```python
from build123d import *

# Parameters (mm, degrees)
F1_DEPTH = 76.2
F2_R     = 3.175
F3_DEPTH = 6.351


with BuildPart() as f1:
    # F0 (on Front) → F1 (new body)
    with BuildSketch(Plane.XZ):
        Polygon((0, 76.2), (0, 0), (42.919317, 0), (42.919317, 6.35), (6.35, 6.35), (6.35, 76.2), align=None)
    extrude(amount=F1_DEPTH)

    # F2 (on face) → F3 (cut, through all)
    with BuildSketch(Plane.XY.offset(6.35)):
        with Locations((24.634659, -19.05)):
            Circle(F2_R)
        with Locations((24.634659, -38.1)):
            Circle(F2_R)
        with Locations((24.634659, -57.15)):
            Circle(F2_R)
    extrude(amount=-F3_DEPTH, mode=Mode.SUBTRACT)


solid = f1.part
```
Can you work these out from the model? Positions are in its coordinate system, mm. A direction names the side the tool comes from. Coordinates: 2 decimals unless noted, no trailing zeros. Loops run counter-clockwise (first coordinate to the right, second up) from the corner with the lowest first, then second, coordinate; pieces in that order, holes last. Notation, with made-up numbers: (37.5, 28) -> (70.5, 28) arc R21 cw to (70.5, 66) -> close; hole circle Ø1 at (39.5, -29.75). An arc over 180 degrees is marked (long way). Put each result on its own line as item: value. Start each with the question number.
Q1. Thinking about a two-plate mould opening in Y: for faces 3 (the face through (5, 0, 30)), 4 (the face through (26.34, -35.42, 3.22)), 5 (the face through (5, -76.2, 30)), which applies, pulls with the +Y half, pulls with the -Y half, needs draft (parallel to the pull), parting line crosses it, or undercut?
Q2. I want a section at B-B (x = 12). Write out the boundary of the cut face in (y, z), plus the area to 3 significant figures.
Q3. For faces 1 (the face through (29, -38, 6.35)), 2 (the face through (26.34, -54.47, 3.22)), which set-ups out of +Z, -Z, +X, -X, +Y, -Y let a thin tool reach every point of the face, with its end or its side?
Q4. I want a section at D-D (y = -18). Write out the boundary of the cut face in (x, z), plus the area to 3 significant figures.
Q5. I want a section at A-A (y = -38.1). Write out the boundary of the cut face in (x, z), plus the area to 3 significant figures.
Q6. I want a section at C-C (y = -50). Write out the boundary of the cut face in (x, z).
Q7. I'm going to push flat-ended pins straight in: P1, Ø3, axis at y = -68, z = 38, coming from the +X side; P2, Ø18.5, axis at x = 29, y = -57, coming from the +Z side. Where does each tip first touch, or does it pass through?
Q8. If I drill on line 1 (X direction, y = -57, z = 2); line 2 (Z direction, x = 13, y = -72.5), over which ranges is the centre line in solid material (lowest first)? Write a range as [from, to].
Taken from the geometry:
1. face 3: pulls with the +Y half
1. face 4: undercut
1. face 5: pulls with the -Y half
2. outline: (-76.2, 0) -> (0, 0) -> (0, 6.35) -> (-76.2, 6.35) -> close
2. area: 484 mm2
3. face 1: +Z, +X, +Y, -Y
3. face 2: +Z, -Z
4. outline: (0, 0) -> (21.64, 0) -> (21.64, 6.35) -> (6.35, 6.35) -> (6.35, 76.2) -> (0, 76.2) -> close; (27.63, 0) -> (42.92, 0) -> (42.92, 6.35) -> (27.63, 6.35) -> close
4. area: 678 mm2
5. outline: (0, 0) -> (21.46, 0) -> (21.46, 6.35) -> (6.35, 6.35) -> (6.35, 76.2) -> (0, 76.2) -> close; (27.81, 0) -> (42.92, 0) -> (42.92, 6.35) -> (27.81, 6.35) -> close
5. area: 676 mm2
6. outline: (0, 0) -> (42.92, 0) -> (42.92, 6.35) -> (6.35, 6.35) -> (6.35, 76.2) -> (0, 76.2) -> close
7. P1: stops at x = 6.35
7. P2: stops at z = 6.35
8. line 1: x = [0, 21.46], [27.81, 42.92]
8. line 2: z = [0, 6.35]
